Part print with two shaded views. Sizes in mm from the minimum x, y, z corner. A direction names the side the tool comes from. Give positions to 0.01 mm unless a question says otherwise; leave off trailing zeros. Write each loop counter-clockwise with the first axis right and the second up, starting at its lowest first coordinate (ties: lowest second). Pieces come first, ordered by that corner, then holes. Notation, with made-up numbers: (29, -22) - (42, -22) arc R24 ccw to (42, 3) - close; hole circle Ø11 at (89.5, 58). An arc over 180 degrees is marked (long way). Answer as a JSON object with one key per item and string values. Group by question number.
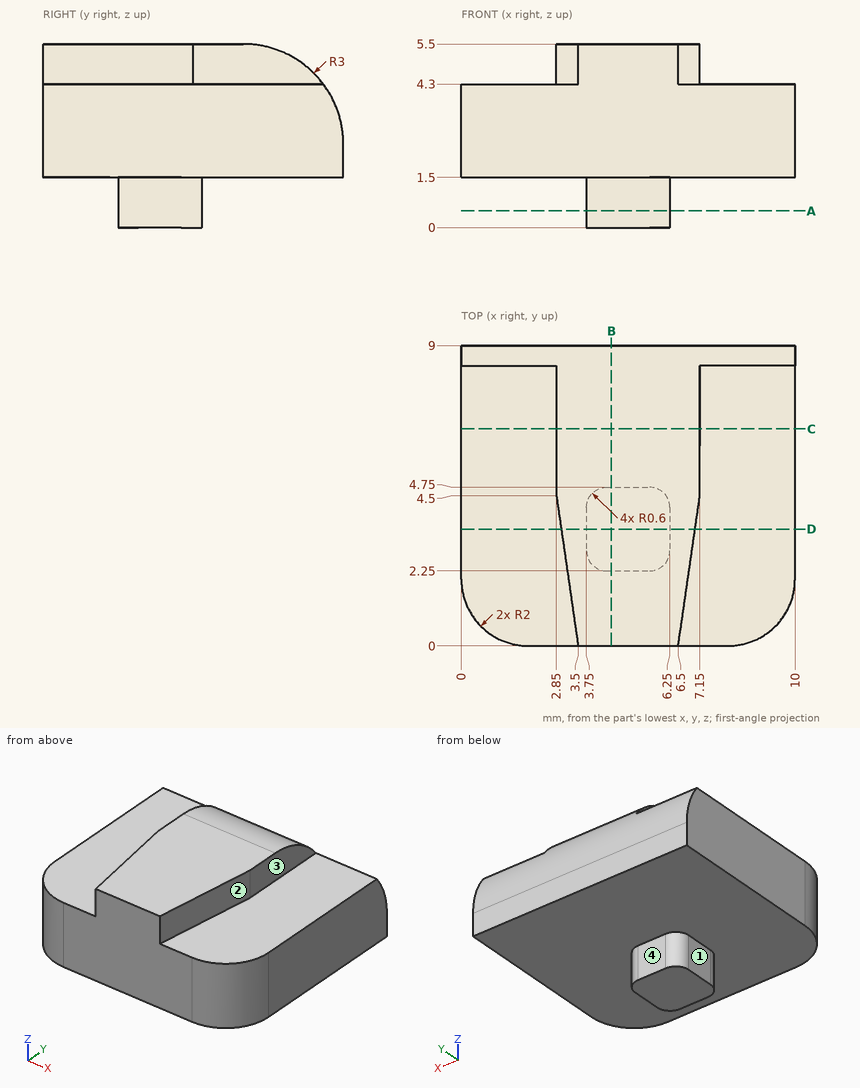
1) Saw through at C-C (y = 6.5). List the corners of the cut face in (x, z), and give its area (3 significant figures).
2) Drop flat-ended pins along their axis: P1, Ø1, axis at x = 1, y = 2.5, coming from the +Z side; P2, Ø1, axis at y = 4, z = 0.5, coming from the +X side; P3, Ø1.5, axis at x = 7, y = 1.5, coming from the +Z side; P4, Ø1.3, axis at y = 7, z = 5, coming from the -X side. Give the stop position or say it passes through.
3) Saw through at A-A (z = 0.5). List the corners of the cut face in (x, y), and give its area (3 significant figures).
4) Which spindle directions (+Z, -Z, +X, -X, +Y, -Y) get a long thin tool onto all of the face, cutting with end or side? Do the marked faces 1, 2, 3 and 4. Say none if no direction does.
5) Saw through at D-D (y = 3.5). List the corners of the cut face in (x, z).
6) Saw through at B-B (x = 4.5). List the corners of the cut face in (y, z).
7) Drill centre lines: line 1 along X through (y, z) = (5.5, 4.5); line 2 along Z through (x, y) = (7.75, 1.5); line 3 along Z through (x, y) = (6.5, 1). Where is each one in solid material? Low to high. Write a range as from..to.
Checks:
{
 "1": {"outline": "(0, 1.5) - (10, 1.5) - (10, 4.3) - (7.15, 4.3) - (7.15, 5.46) - (2.85, 5.46) - (2.85, 4.3) - (0, 4.3) - close", "area": "33.0 mm2"},
 "2": {"P1": "z = 4.3", "P2": "x = 6.25", "P3": "z = 5.5", "P4": "x = 2.85"},
 "3": {"outline": "(3.75, 2.85) arc R0.6 ccw to (4.35, 2.25) - (5.65, 2.25) arc R0.6 ccw to (6.25, 2.85) - (6.25, 4.15) arc R0.6 ccw to (5.65, 4.75) - (4.35, 4.75) arc R0.6 ccw to (3.75, 4.15) - close", "area": "5.94 mm2"},
 "4": {"face 1": "-Z, -X, +Y, -Y", "face 2": "+Z, +X, -Y", "face 3": "+Z, +X, +Y, -Y", "face 4": "-Z, +X, -X, +Y"},
 "5": {"outline": "(0, 1.5) - (3.75, 1.5) - (3.75, 0) - (6.25, 0) - (6.25, 1.5) - (10, 1.5) - (10, 4.3) - (7.01, 4.3) - (7.01, 5.5) - (2.99, 5.5) - (2.99, 4.3) - (0, 4.3) - close"},
 "6": {"outline": "(0, 1.5) - (2.25, 1.5) - (2.25, 0) - (4.75, 0) - (4.75, 1.5) - (9, 1.5) - (9, 2.5) arc R3 ccw to (6, 5.5) - (0, 5.5) - close"},
 "7": {"line 1": "2.85..7.15", "line 2": "1.5..4.3", "line 3": "1.5..5.5"}
}
